from build123d import *

# Parameters (mm, degrees)
MAINSHAPE_DEPTH = 3.175
FILLET1_R       = 12.7


with BuildPart() as part:
    # Sketch1 → MainShape (new body)
    with BuildSketch(Plane.XY):
        Polygon((0, 0), (63.5, 127), (114.3, 127), (177.8, 0), align=None)
    extrude(amount=MAINSHAPE_DEPTH)

    # Fillet1
    fillet1_edges = [part.edges().sort_by_distance(p)[0] for p in [
        (63.5, 127, 1.5875),
        (114.3, 127, 1.5875),
    ]]
    fillet(fillet1_edges, radius=FILLET1_R)


solid = part.part
Could you check a few things on this model? Use its own coordinates, in mm. Give positions to 0.01 mm unless a question says otherwise; leave off trailing zeros. Order: outer loops, then holes, each group sorted by start corner. A loop starts at its lowest first (then second) coordinate and runs counter-clockwise, first axis right, second up.
Item 1: If we section it at B-B, the plane y = 114: Write out the boundary of the cut face in (x, z) (3 decimals), plus the area to 3 significant figures.
Item 2: If we section it at C-C, the plane x = 165.5: Write out the boundary of the cut face in (y, z) (3 decimals).
Item 3: I need wall thicknesses on line 1 (X direction, y = 14, z = 2.9); line 2 (X direction, y = 98, z = 1.4); line 3 (Y direction, x = 28, z = 2.35). Which ranges of each line are inside material? Lowest first, please.
Item 4: If we section it at A-A, the plane z = 0.8: Write out the boundary of the cut face in (x, y), plus the area to 3 significant figures.
Values:
1. outline: (57, 0) - (120.8, 0) - (120.8, 3.175) - (57, 3.175) - close
1. area: 203 mm2
2. outline: (0, 0) - (24.6, 0) - (24.6, 3.175) - (0, 3.175) - close
3. line 1: x = 7 to 170.8
3. line 2: x = 49 to 128.8
3. line 3: y = 0 to 56
4. outline: (0, 0) - (177.8, 0) - (117.81, 119.98) arc R12.7 ccw to (106.45, 127) - (71.35, 127) arc R12.7 ccw to (59.99, 119.98) - close
4. area: 14,500 mm2
